Autodesk Inventor part; units mm, degrees
ref_plane "YZ Plane" through (0, 0, 0) normal (1, 0, 0) x (0, 1, 0)
ref_plane "XZ Plane" through (0, 0, 0) normal (0, 1, 0) x (-1, 0, 0)
ref_plane "XY Plane" through (0, 0, 0) normal (0, 0, 1) x (1, 0, 0)
sketch "Sketch1" plane through (0, 0, 0) normal (0, 1, 0) x (-1, 0, 0)
  circle A0 centre (-92.5739, -114.0841) radius 1.75
  line L0 (-104.8331, -105.8291) -> (-88.5698, -105.8291)
  line L1 (-88.5698, -105.8291) -> (-88.5698, -122.3391)
  line L2 (-88.5698, -122.3391) -> (-104.8331, -122.3391)
  line L3 (-104.8331, -105.8291) -> (-121.0891, -105.8291)
  line L4 (-121.0891, -105.8291) -> (-121.0891, -122.3391)
  line L5 (-121.0891, -122.3391) -> (-104.8331, -122.3391)
  circle A1 centre (-117.0886, -114.0841) radius 1.75
  point P0 (0, 0)
  point P1 (0, 0)
extrude "Extrusion1" add sketch "Sketch1" along normal blind 5.588
sketch "Sketch2" plane through (88.5698, 0, -105.8291) normal (0, 0, 1) x (1, 0, 0)
  line L0 (0, 5.588) -> (32.5193, 5.588)
  line L1 (0, 5.588) -> (32.5193, 5.588)
  arc A0 (8.0046, -7.239) -> (24.5146, -7.239) centre (16.2596, -7.239) ccw
  line L2 (8.0046, -7.239) -> (8.0046, 0)
  line L3 (0, 0) -> (32.5193, 0)
  line L4 (8.0046, 0) -> (24.5146, 0)
  line L5 (24.5146, 0) -> (24.5146, -7.239)
  circle A1 centre (16.2596, -7.2898) radius 3.9688
  point P0 (-88.5698, 0)
  dimension "d14" = 7.9375
fillet "Fillet2" radius 3.175 4 edges at (88.5698, 2.794, -122.3391) (88.5698, 2.794, -105.8291) (121.0891, 2.794, -122.3391) (121.0891, 2.794, -105.8291)
extrude "Extrusion3" add sketch "Sketch2" against normal blind 16.51
fillet "Fillet3" radius 1.27 2 edges at (96.5744, 0, -114.0841) (113.0844, 0, -114.0841)
chamfer "Chamfer2" distance 0.635 angle 45 2 edges at (100.8607, -7.2898, -105.8291) (100.8607, -7.2898, -122.3391)
properties part number "shaftMount"
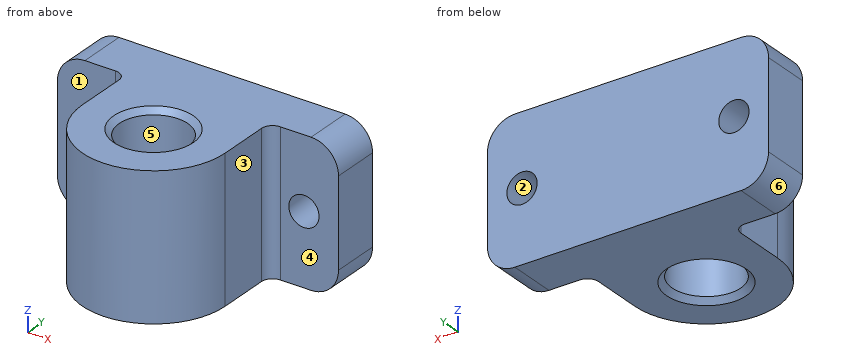
Geometry check sheet. Reference: the model listing, model coordinates, mm. Face numbers are marked on the shaded views. A direction names the side the tool comes from. Coordinates: 2 decimals unless noted, no trailing zeros. Order: outer loops, then holes, each group sorted by start corner. A loop starts at its lowest first (then second) coordinate and runs counter-clockwise, first axis right, second up.
Item 1: Depth check by flat-ended pin: pin 1 (3 mm diameter, centred on x = 92.57, z = -114.08, fed in from -Y); pin 2 (6 mm diameter, centred on y = -3.5, z = -120.5, fed in from +X); pin 3 (3.5 mm diameter, centred on x = 91.5, z = -115.5, fed in from -Y); pin 4 (1.8 mm diameter, centred on y = -3, z = -116.5, fed in from -X). Enter the tip coordinate at first touch or a pass-through.
Item 2: Section check B-B (z = -114.5). Enter the section's corners in (x, y) (3 decimals).
Item 3: Tool access check on the marked faces 1, 2 and 3. Record the directions out of +Z, -Z, +X, -X, +Y, -Y that give a thin tool (end or side, any length) a straight path to the whole face; none if there is none.
Item 4: Mould release check, pull along Y, two halves, no side actions. Record for the marked faces 4, 5 and 6: released by +Y, released by -Y, zero draft, split by the parting line, or undercut.
Item 5: Scan lines: line 1 along X through (y, z) = (-1.75, -119.75); line 2 along X through (y, z) = (4.25, -113); line 3 along X through (y, z) = (-4, -111.5). Record each from-to range of solid material in increasing order.
Item 6: Section check A-A (x = 92.5). Enter the section's corners in (y, z).
Item 7: Section check D-D (z = -110.5). Enter the section's corners in (x, y) (3 decimals).
Item 8: Section check C-C (y = 3.5). Enter the section's corners in (x, z) (3 decimals).
Check sheet entries:
1. pin 1: passes through
1. pin 2: stops at x = 113.34
1. pin 3: stops at y = 0
1. pin 4: stops at x = 96.57
2. outline: (88.57, 0) - (90.874, 0) - (90.874, 5.588) - (88.57, 5.588) - close; (94.274, 0) - (95.304, 0) arc R1.27 cw to (96.574, -1.27) - (96.574, -7.239) arc R8.255 ccw to (113.084, -7.239) - (113.084, -1.27) arc R1.27 cw to (114.354, 0) - (115.389, 0) - (115.389, 5.588) - (94.274, 5.588) - close; (118.788, 0) - (121.089, 0) - (121.089, 5.588) - (118.788, 5.588) - close; hole circle Ø7.938 at (104.829, -7.29)
3. face 1: +Z, -Z, -X, -Y
3. face 2: +Y, -Y
3. face 3: +Z, -Z, +X, -Y
4. face 4: released by -Y
4. face 5: undercut
4. face 6: zero draft
5. line 1: x = 96.57 to 113.08
5. line 2: x = 88.57 to 91.2, 93.95 to 115.71, 118.46 to 121.09
5. line 3: x = 96.57 to 102.61, 107.05 to 113.08
6. outline: (0, -122.34) - (5.59, -122.34) - (5.59, -115.83) - (0, -115.83) - close; (0, -112.34) - (5.59, -112.34) - (5.59, -105.83) - (0, -105.83) - close
7. outline: (88.57, 0) - (95.304, 0) arc R1.27 cw to (96.574, -1.27) - (96.574, -7.239) arc R8.255 ccw to (113.084, -7.239) - (113.084, -1.27) arc R1.27 cw to (114.354, 0) - (121.089, 0) - (121.089, 5.588) - (88.57, 5.588) - close; hole circle Ø7.938 at (104.829, -7.29)
8. outline: (88.57, -119.164) arc R3.175 ccw to (91.745, -122.339) - (117.914, -122.339) arc R3.175 ccw to (121.089, -119.164) - (121.089, -109.004) arc R3.175 ccw to (117.914, -105.829) - (91.745, -105.829) arc R3.175 ccw to (88.57, -109.004) - close; hole circle Ø3.5 at (92.574, -114.084); hole circle Ø3.5 at (117.089, -114.084)
